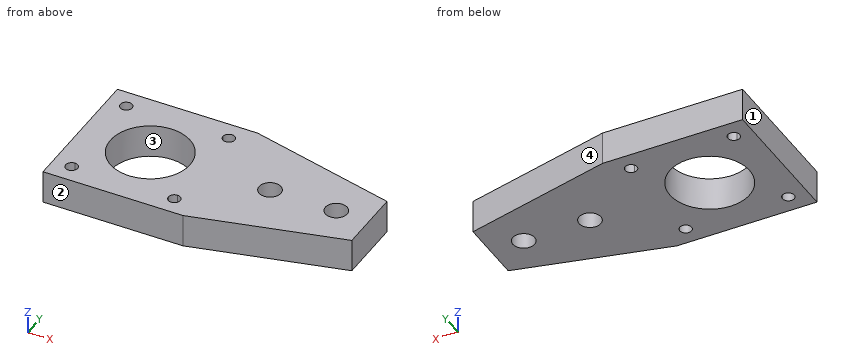
```python
from build123d import *

# Parameters (mm, degrees)
F0_W     = 45
F0_H     = 20
F0_R     = 3.3
F0_R_2   = 12
F1_DEPTH = 10


with BuildPart() as f1:
    # F0 (on Top) → F1 (new body)
    with BuildSketch(Plane.XY):
        with Locations((43.65, 0)):
            Rectangle(F0_W, F0_H)
        with Locations((36.15, 0)):
            Circle(F0_R, mode=Mode.SUBTRACT)
        with Locations((56.15, 0)):
            Circle(F0_R, mode=Mode.SUBTRACT)
        Polygon((66.15, 10), (21.15, 21.15), (21.15, 10), align=None)
        Polygon((66.15, -10), (21.15, -10), (21.15, -21.15), align=None)
        Polygon((21.15, 10), (21.15, 21.15), (-21.15, 21.15), (-21.15, -21.15), (21.15, -21.15), (21.15, -10), align=None)
        with BuildLine():
            ThreePointArc((-15.5, 13.7), (-16.772792, 16.772792), (-13.7, 15.5))
            Line((-13.7, 15.5), (13.7, 15.5))
            ThreePointArc((13.7, 15.5), (15.5, 17.3), (17.3, 15.5))
            ThreePointArc((17.3, 15.5), (16.772792, 14.227208), (15.5, 13.7))
            Line((15.5, 13.7), (15.5, -13.7))
            ThreePointArc((15.5, -13.7), (16.772792, -14.227208), (17.3, -15.5))
            ThreePointArc((17.3, -15.5), (15.5, -17.3), (13.7, -15.5))
            Line((13.7, -15.5), (-13.7, -15.5))
            ThreePointArc((-13.7, -15.5), (-16.772792, -16.772792), (-15.5, -13.7))
            Line((-15.5, -13.7), (-15.5, 13.7))
        make_face(mode=Mode.SUBTRACT)
        with BuildLine():
            Line((13.7, 15.5), (-13.7, 15.5))
            ThreePointArc((-13.7, 15.5), (-14.227208, 14.227208), (-15.5, 13.7))
            Line((-15.5, 13.7), (-15.5, -13.7))
            ThreePointArc((-15.5, -13.7), (-14.227208, -14.227208), (-13.7, -15.5))
            Line((-13.7, -15.5), (13.7, -15.5))
            ThreePointArc((13.7, -15.5), (14.227208, -14.227208), (15.5, -13.7))
            Line((15.5, -13.7), (15.5, 13.7))
            ThreePointArc((15.5, 13.7), (14.227208, 14.227208), (13.7, 15.5))
        make_face()
        Circle(F0_R_2, mode=Mode.SUBTRACT)
    extrude(amount=F1_DEPTH)


solid = f1.part
```
The model under review builds one solid part; all positions refer to its coordinate system, in mm. Face numbers are marked on the shaded views. Round coordinates to 2 decimals unless told otherwise and drop trailing zeros. Order: outer loops, then holes, each group sorted by start corner. A loop starts at its lowest first (then second) coordinate and runs counter-clockwise, first axis right, second up. Notation, with made-up numbers: (-8.5, -21) - (20.5, -21) arc R9 ccw to (20.5, -17) - close; hole circle Ø4 at (-5.75, -38). An arc over 180 degrees is marked (long way). Answer in a Markdown table with one row per item.
(1) Take a section at A-A on z = 6.5. Write out the cut boundary in (x, y).
Result set:
| item | result |
|---|---|
| outline | (-21.15, -21.15) - (21.15, -21.15) - (66.15, -10) - (66.15, 10) - (21.15, 21.15) - (-21.15, 21.15) - close; hole circle Ø3.6 at (-15.5, -15.5); hole circle Ø3.6 at (-15.5, 15.5); hole circle Ø24 at (0, 0); hole (13.7, -15.5) arc R1.8 ccw (long way) to (15.5, -13.7) arc R1.8 ccw to start; hole (15.5, 13.7) arc R1.8 ccw to (17.3, 15.5) arc R1.8 ccw (long way) to start; hole circle Ø6.6 at (36.15, 0); hole circle Ø6.6 at (56.15, 0) |
(2) Take a section at D-D on x = 54. Write out the cut boundary in (y, z), plus the area to 3 significant figures.
Result set:
| item | result |
|---|---|
| outline | (-13.01, 0) - (-2.5, 0) - (-2.5, 10) - (-13.01, 10) - close; (2.5, 0) - (13.01, 0) - (13.01, 10) - (2.5, 10) - close |
| area | 210 mm2 |
(3) Mouldability with a two-part tool opening along X and no side actions: class the marked faces 1, 2, 3 and 4 as released by +X, released by -X, zero draft, split by the parting line, or undercut.
Result set:
| item | result |
|---|---|
| face 1 | released by -X |
| face 2 | zero draft |
| face 3 | undercut |
| face 4 | released by +X |
(4) Take a section at B-B on y = 0. Write out the cut boundary in (x, z), plus the area to 3 significant figures.
Result set:
| item | result |
|---|---|
| outline | (-21.15, 0) - (-12, 0) - (-12, 10) - (-21.15, 10) - close; (12, 0) - (32.85, 0) - (32.85, 10) - (12, 10) - close; (39.45, 0) - (52.85, 0) - (52.85, 10) - (39.45, 10) - close; (59.45, 0) - (66.15, 0) - (66.15, 10) - (59.45, 10) - close |
| area | 501 mm2 |
(5) For line 1 (Y direction, x = -15.5, z = 2.5); line 2 (Y direction, x = -14.5, z = 5.75); line 3 (Y direction, x = 0, z = 5), list the stretches that pass through material, from the lowest coordinate up. Write a range as from..to.
Result set:
| item | result |
|---|---|
| line 1 | y = -21.15..-17.3, -13.7..13.7, 17.3..21.15 |
| line 2 | y = -21.15..-17, -14..14, 17..21.15 |
| line 3 | y = -21.15..-12, 12..21.15 |
(6) Take a section at C-C on x = 0. Write out the cut boundary in (y, z).
Result set:
| item | result |
|---|---|
| outline | (-21.15, 0) - (-12, 0) - (-12, 10) - (-21.15, 10) - close; (12, 0) - (21.15, 0) - (21.15, 10) - (12, 10) - close |
